from build123d import *

# Parameters (mm, degrees)
BOSS_EXTRUDE6_DEPTH = 42
SKETCH9_W           = 42
SKETCH9_H           = 14
BOSS_EXTRUDE7_DEPTH = 3
SKETCH10_W          = 62
SKETCH10_H          = 3
BOSS_EXTRUDE8_DEPTH = 17
SKETCH11_R          = 1.75
SKETCH11_R_2        = 14
CUT_EXTRUDE3_DEPTH  = 4
SKETCH12_R          = 2.25
CUT_EXTRUDE4_DEPTH  = 4


with BuildPart() as part:
    # Sketch7 → Boss-Extrude6 (new body)
    with BuildSketch(Plane.XY):
        Polygon((42, -17), (62, -17), (62, -14), (45, -14), (45, 0), (0, 0), (0, -3), (42, -3), align=None)
    extrude(amount=BOSS_EXTRUDE6_DEPTH)

    # Sketch9 → Boss-Extrude7 (add)
    with BuildSketch(Plane.XY.offset(42)):
        with Locations((21, -10)):
            Rectangle(SKETCH9_W, SKETCH9_H)
        Polygon((45, -14), (45, 0), (0, 0), (0, -3), (42, -3), (42, -17), (62, -17), (62, -14), align=None)
    extrude(amount=BOSS_EXTRUDE7_DEPTH)

    # Sketch10 → Boss-Extrude8 (add)
    with BuildSketch(Plane.XY.offset(45)):
        with Locations((31, -15.5)):
            Rectangle(SKETCH10_W, SKETCH10_H)
    extrude(amount=BOSS_EXTRUDE8_DEPTH)

    # Sketch11 → Cut-Extrude3 (cut, through all)
    with BuildSketch(Plane.XZ.offset(3)):
        with Locations((5.5, 36.5)):
            Circle(SKETCH11_R)
        with Locations((36.5, 36.5)):
            Circle(SKETCH11_R)
        with Locations((36.5, 5.5)):
            Circle(SKETCH11_R)
        with Locations((5.5, 5.5)):
            Circle(SKETCH11_R)
        with Locations((21, 21)):
            Circle(SKETCH11_R_2)
    extrude(amount=-CUT_EXTRUDE3_DEPTH, mode=Mode.SUBTRACT)

    # Sketch12 → Cut-Extrude4 (cut, through all)
    with BuildSketch(Plane(origin=(0, -14, 0), x_dir=(1, 0, 0), z_dir=(0, 1, 0))):
        with Locations((11.25, -53.5)):
            Circle(SKETCH12_R)
        with Locations((33.75, -53.5)):
            Circle(SKETCH12_R)
        with Locations((53.5, -53.5)):
            Circle(SKETCH12_R)
        with Locations((53.5, -11.25)):
            Circle(SKETCH12_R)
        with Locations((53.5, -33.75)):
            Circle(SKETCH12_R)
    extrude(amount=-CUT_EXTRUDE4_DEPTH, mode=Mode.SUBTRACT)


solid = part.part
Check sheet for the modelled part. Datum: model origin and axes. Units: mm. A direction names the side the tool comes from. Round coordinates to 2 decimals unless told otherwise and drop trailing zeros. Loops run counter-clockwise (first coordinate to the right, second up) from the corner with the lowest first, then second, coordinate; pieces in that order, holes last. Notation, with made-up numbers: M 35.5,13 L 83.5,13 A35 ccw 83.5,49 Z; hole C 74.25,85.25 d9. An arc over 180 degrees is marked long. One line per item, written item: value.
(1) Sectioned sample at A-A, the plane z = 53.5. Record the cut outline in (x, y).
Computed values:
outline: M 0,-17 L 9,-17 L 9,-14 L 0,-14 Z; M 13.5,-17 L 31.5,-17 L 31.5,-14 L 13.5,-14 Z; M 36,-17 L 51.25,-17 L 51.25,-14 L 36,-14 Z; M 55.75,-17 L 62,-17 L 62,-14 L 55.75,-14 Z
(2) Access from +Z, -Z, +X, -X, +Y, -Y to the whole of each face (thin tool, end or side, straight path). Record for faces 5 (the face through (22, -7, 45)), 6 (the face through (42, -10, 21)), 7 (the face through (45, -7, 22)).
Computed values:
face 5: +Z, +X, -X, +Y
face 6: -Z, -X, -Y
face 7: +Z, -Z, +X, +Y
(3) Depth check by flat-ended pin: pin 1 Ø3 at (y, z) = (-7.5, 15.5) entering from +X; pin 2 Ø4 at (y, z) = (-10.5, 20) entering from -X; pin 3 Ø5.5 at (x, z) = (36.5, 36.5) entering from -Y. Enter the tip coordinate at first touch or a pass-through.
Computed values:
pin 1: stops at x = 45
pin 2: stops at x = 42
pin 3: stops at y = -3
(4) Sectioned sample at B-B, the plane z = 5.5. Record the cut outline in (x, y), then the cut area to 3 significant figures.
Computed values:
outline: M 0,-3 L 3.75,-3 L 3.75,0 L 0,0 Z; M 7.25,-3 L 34.75,-3 L 34.75,0 L 7.25,0 Z; M 38.25,-3 L 42,-3 L 42,-17 L 62,-17 L 62,-14 L 45,-14 L 45,0 L 38.25,0 Z
area: 207 mm^2
(5) Sectioned sample at C-C, the plane x = 53.5. Record the cut outline in (y, z).
Computed values:
outline: M -17,0 L -14,0 L -14,9 L -17,9 Z; M -17,13.5 L -14,13.5 L -14,31.5 L -17,31.5 Z; M -17,36 L -14,36 L -14,51.25 L -17,51.25 Z; M -17,55.75 L -14,55.75 L -14,62 L -17,62 Z
(6) Release check for a two-part mould opening along Z. For faces 1 (the face through (6.7, -3, 20.7)), 2 (the face through (5.12, -1.52, 3.79)), 3 (the face through (21, -10, 42)), 4 (the face through (34.96, -15.479, 51.603)) record: +Z half, -Z half, draft (parallel to the pull), parting line (faces both ways), or undercut.
Computed values:
face 1: draft
face 2: undercut
face 3: -Z half
face 4: undercut
(7) Sectioned sample at D-D, the plane x = 5.5. Record the cut outline in (y, z).
Computed values:
outline: M -17,42 L -3,42 L -3,38.25 L 0,38.25 L 0,45 L -14,45 L -14,62 L -17,62 Z; M -3,0 L 0,0 L 0,3.75 L -3,3.75 Z; M -3,7.25 L 0,7.25 L 0,34.75 L -3,34.75 Z
(8) Thickness scan on line 1 (Z direction, x = 36.5, y = -2.2); line 2 (X direction, y = -15.3, z = 53.5); line 3 (Z direction, x = 21, y = -1.5). Record the ranges inside material, lowest first.
Computed values:
line 1: z = 0 to 3.75, 7.25 to 34.75, 38.25 to 45
line 2: x = 0 to 9, 13.5 to 31.5, 36 to 51.25, 55.75 to 62
line 3: z = 0 to 7, 35 to 45
